Could you check a few things on this model? Use its own coordinates, in mm. A direction names the side the tool comes from. Give positions to 0.01 mm unless a question says otherwise; leave off trailing zeros. Order: outer loops, then holes, each group sorted by start corner. A loop starts at its lowest first (then second) coordinate and runs counter-clockwise, first axis right, second up. Notation, with made-up numbers: (64, 64) -> (70, 64) arc R22 ccw to (70, 75) -> close; hole circle Ø10 at (61, -30.75). An arc over 180 degrees is marked (long way). One line per item, written item: value.
```python
from build123d import *

# Parameters (mm, degrees)
SKETCH1_W           = 140
SKETCH1_H           = 90
BOSS_EXTRUDE1_DEPTH = 3
SKETCH2_W           = 4
SKETCH2_H           = 1.5
BOSS_EXTRUDE2_DEPTH = 20
SKETCH4_W           = 55.5
SKETCH4_H           = 40.7
CUT_EXTRUDE1_DEPTH  = 1.5


with BuildPart() as part:
    # Sketch1 → Boss-Extrude1 (new body)
    with BuildSketch(Plane(origin=(0, 0, 0), x_dir=(0, 1, 0), z_dir=(0, 0, 1))):
        Rectangle(SKETCH1_W, SKETCH1_H)
    extrude(amount=BOSS_EXTRUDE1_DEPTH)

    # Sketch2 → Boss-Extrude2 (add)
    with BuildSketch(Plane.XY.offset(3)):
        with Locations((-43, 69.25)):
            Rectangle(SKETCH2_W, SKETCH2_H)
        with Locations((-15.6, 69.25)):
            Rectangle(SKETCH2_W, SKETCH2_H)
        with Locations((15.6, 69.25)):
            Rectangle(SKETCH2_W, SKETCH2_H)
        with Locations((43, 69.25)):
            Rectangle(SKETCH2_W, SKETCH2_H)
        with Locations((-43, -69.25)):
            Rectangle(SKETCH2_W, SKETCH2_H)
        with Locations((-15.6, -69.25)):
            Rectangle(SKETCH2_W, SKETCH2_H)
        with Locations((15.6, -69.25)):
            Rectangle(SKETCH2_W, SKETCH2_H)
        with Locations((43, -69.25)):
            Rectangle(SKETCH2_W, SKETCH2_H)
    extrude(amount=BOSS_EXTRUDE2_DEPTH)

    # Sketch4 → Cut-Extrude1 (cut)
    with BuildSketch(Plane.XY.offset(3)):
        Rectangle(SKETCH4_W, SKETCH4_H)
    extrude(amount=-CUT_EXTRUDE1_DEPTH, mode=Mode.SUBTRACT)


solid = part.part
```
1) Suppose I cut it at C-C, the plane x = -5. Write out the boundary of the cut face in (y, z).
Answer below:
outline: (-70, 0) -> (70, 0) -> (70, 3) -> (20.35, 3) -> (20.35, 1.5) -> (-20.35, 1.5) -> (-20.35, 3) -> (-70, 3) -> close
2) For P1, Ø1.5, axis at x = 7.5, y = 4.5, coming from the +Z side; P2, Ø12, axis at x = -25, y = 42.5, coming from the +Z side, each with a flat end and sliding along its axis, tell me the tip position at first contact or that it passes through.
Answer below:
P1: stops at z = 1.5
P2: stops at z = 3
3) Suppose I cut it at B-B, the plane y = 11. Write out the boundary of the cut face in (x, z).
Answer below:
outline: (-45, 0) -> (45, 0) -> (45, 3) -> (27.75, 3) -> (27.75, 1.5) -> (-27.75, 1.5) -> (-27.75, 3) -> (-45, 3) -> close
4) Suppose I cut it at D-D, the plane y = 52. Write out the boundary of the cut face in (x, z), then the cut area to 3 significant figures.
Answer below:
outline: (-45, 0) -> (45, 0) -> (45, 3) -> (-45, 3) -> close
area: 270 mm2
5) We'd pull the mould along X, two halves only. Please class faces 3 (the flat face through (0, 70, 1)), 4 (the flat face through (45, 0, 1)), 5 (the flat face through (-45, 0, 1)), 6 (the flat face through (0, 0, 1.5)): +X half, -X half, draft (parallel to the pull), parting line (faces both ways), or undercut.
Answer below:
face 3: draft
face 4: +X half
face 5: -X half
face 6: undercut
6) For faces 1 (the flat face through (-43, 68.5, 13)), 2 (the flat face through (-1, -1, 0)), which set-ups out of +Z, -Z, +X, -X, +Y, -Y let a thin tool reach every point of the face, with its end or its side?
Answer below:
face 1: +Z, +X, -X
face 2: -Z, +X, -X, +Y, -Y
7) If I drill on line 1 along X through (y, z) = (-12, 1.75); line 2 along Y through (x, z) = (-7.5, 2); line 3 along Z through (x, y) = (31.5, 11), over which ranges is the centre line in solid material (lowest first)?
Answer below:
line 1: x = -45 to -27.75, 27.75 to 45
line 2: y = -70 to -20.35, 20.35 to 70
line 3: z = 0 to 3
8) Suppose I cut it at A-A, the plane z = 18.25. State how many separate pieces and enclosed holes the cut face has, then the cut area to 3 significant figures.
Answer below:
separate pieces: 8
enclosed holes: 0
area: 48.0 mm2
